Geometry: final body of the model. Coordinates: model frame, mm. A direction names the side the tool comes from. Round coordinates to 2 decimals unless told otherwise and drop trailing zeros. Loops run counter-clockwise (first coordinate to the right, second up) from the corner with the lowest first, then second, coordinate; pieces in that order, holes last. Notation, with made-up numbers: (84.25, 10.5) - (134.25, 10.5) arc R27 ccw to (134.25, 37.5) - close; hole circle Ø2 at (9.25, 5.25). An arc over 180 degrees is marked (long way). Return JSON: item names as keys, results as strings. Group by question number.
1. Section D-D on z = 3.75. Return loops of the section in (x, y), and give its area (3 significant figures).
2. Draft query along Z for faces 1 (the face through (-17.465, -0.338, 24.578)), 2 (the face through (15, 0, 17)), 3 (the face through (-17, -7, 29)). Return one class per face: +Z half, -Z half, draft (parallel to the pull), parting line (faces both ways), or undercut.
3. Section B-B on y = 1.5. Return loops of the section in (x, z).
4. First-contact query: pin 1 Ø3 at (x, y) = (-10, 0) entering from -Z (3 decimals); pin 2 Ø1 at (x, y) = (-9, -3) entering from +Z. Flat tips, straight axial feed; report the tip coordinate or a pass-through.
5. Section C-C on x = 18. Return loops of the section in (y, z).
6. Material intervals for probe 1 along X at (y, z) = (-4.5, 11.5); probe 2 along Y at (x, z) = (-10, 1.35); probe 3 along Z at (x, y) = (-16.95, 0), sorted ascending.
7. Set-up query: faces 4 (the face through (-7.52, 0.78, 2.46)), 5 (the face through (0, 0, 5)). Return all of +Z, -Z, +X, -X, +Y, -Y with unobstructed straight access to the full face (end or side cutting, diameter ignored); none if empty.
8. Section A-A on x = 10. Return loops of the section in (y, z).
from build123d import *

# Parameters (mm, degrees)
SKETCH_W     = 40
SKETCH_H     = 18
SKETCH_R     = 2.6
PAD_DEPTH    = 5
SKETCH001_W  = 5
SKETCH001_H  = 18
PAD001_DEPTH = 25
SKETCH002_R  = 2.6
POCKET_DEPTH = 40.001
FILLET_R     = 5


with BuildPart() as part:
    # Sketch → Pad (new body)
    with BuildSketch(Plane.XY):
        Rectangle(SKETCH_W, SKETCH_H)
        with Locations((10, 0)):
            Circle(SKETCH_R, mode=Mode.SUBTRACT)
        with Locations((-10, 0)):
            Circle(SKETCH_R, mode=Mode.SUBTRACT)
    extrude(amount=PAD_DEPTH)

    # Sketch001 (on Face8 of Pad) → Pad001 (join)
    with BuildSketch(Plane.XY.offset(5)):
        with Locations((-17.5, 0)):
            Rectangle(SKETCH001_W, SKETCH001_H)
        with Locations((17.5, 0)):
            Rectangle(SKETCH001_W, SKETCH001_H)
    extrude(amount=PAD001_DEPTH)

    # Sketch002 (on Face15 of Pad001) → Pocket (cut, through all)
    with BuildSketch(Plane.YZ.offset(20)):
        with Locations((0, 22)):
            Circle(SKETCH002_R)
    extrude(amount=-POCKET_DEPTH, mode=Mode.SUBTRACT)

    # Fillet
    fillet_edges = [part.edges().sort_by_distance(p)[0] for p in [
        (17.5, -9, 30),
        (17.5, 9, 30),
        (-17.5, 9, 30),
        (-17.5, -9, 30),
    ]]
    fillet(fillet_edges, radius=FILLET_R)


solid = part.part
Taken from the geometry:
{
 "1": {"outline": "(-20, -9) - (20, -9) - (20, 9) - (-20, 9) - close; hole circle Ø5.2 at (-10, 0); hole circle Ø5.2 at (10, 0)", "area": "678 mm2"},
 "2": {"face 1": "undercut", "face 2": "draft", "face 3": "+Z half"},
 "3": {"outline": "(-20, 0) - (-12.12, 0) - (-12.12, 5) - (-15, 5) - (-15, 19.88) - (-20, 19.88) - close; (-20, 24.12) - (-15, 24.12) - (-15, 30) - (-20, 30) - close; (-7.88, 0) - (7.88, 0) - (7.88, 5) - (-7.88, 5) - close; (12.12, 0) - (20, 0) - (20, 19.88) - (15, 19.88) - (15, 5) - (12.12, 5) - close; (15, 24.12) - (20, 24.12) - (20, 30) - (15, 30) - close"},
 "4": {"pin 1": "through", "pin 2": "z = 5"},
 "5": {"outline": "(-9, 0) - (9, 0) - (9, 25) arc R5 ccw to (4, 30) - (-4, 30) arc R5 ccw to (-9, 25) - close; hole circle Ø5.2 at (0, 22)"},
 "6": {"probe 1": "-20 to -15, 15 to 20", "probe 2": "-9 to -2.6, 2.6 to 9", "probe 3": "0 to 19.4, 24.6 to 30"},
 "7": {"face 4": "+Z, -Z", "face 5": "+Z, +Y, -Y"},
 "8": {"outline": "(-9, 0) - (-2.6, 0) - (-2.6, 5) - (-9, 5) - close; (2.6, 0) - (9, 0) - (9, 5) - (2.6, 5) - close"}
}
